Here's the drawing with two shaded views (mm, measured from the low corner). I have some questions. Coordinates: 2 decimals unless noted, no trailing zeros. Loops run counter-clockwise (first coordinate to the right, second up) from the corner with the lowest first, then second, coordinate; pieces in that order, holes last.
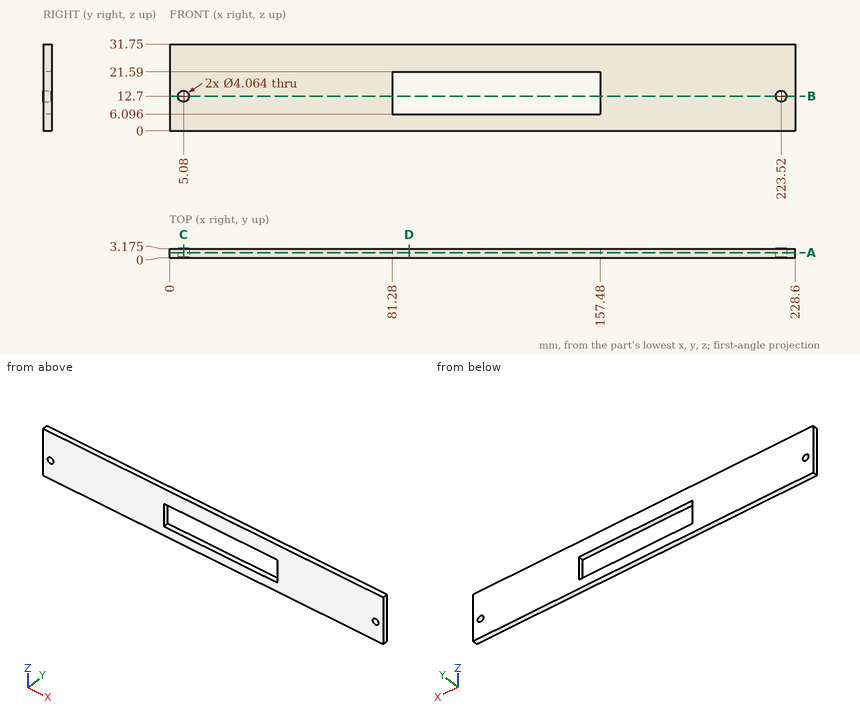
(1) I want a section at C-C on x = 5.08. Write out the boundary of the cut face in (y, z) (3 decimals).
Check values:
outline: (0, 0) - (3.175, 0) - (3.175, 10.668) - (0, 10.668) - close; (0, 14.732) - (3.175, 14.732) - (3.175, 31.75) - (0, 31.75) - close
(2) If I drill on probe 1 along X at (y, z) = (1.8, 12.7); probe 2 along Z at (x, y) = (223.52, 1.5); probe 3 along X at (y, z) = (2.6, 12.5), over which ranges is the centre line in solid material (lowest first)?
Check values:
probe 1: x = 0 to 3.05, 7.11 to 81.28, 157.48 to 221.49, 225.55 to 228.6
probe 2: z = 0 to 10.67, 14.73 to 31.75
probe 3: x = 0 to 3.06, 7.1 to 81.28, 157.48 to 221.5, 225.54 to 228.6
(3) I want a section at D-D on x = 87.5. Write out the boundary of the cut face in (y, z) (3 decimals), then the cut area to 3 significant figures.
Check values:
outline: (0, 0) - (3.175, 0) - (3.175, 6.096) - (0, 6.096) - close; (0, 21.59) - (3.175, 21.59) - (3.175, 31.75) - (0, 31.75) - close
area: 51.6 mm2
(4) I want a section at B-B on z = 12.7. Write out the boundary of the cut face in (x, y) (3 decimals).
Check values:
outline: (0, 0) - (3.048, 0) - (3.048, 3.175) - (0, 3.175) - close; (7.112, 0) - (81.28, 0) - (81.28, 3.175) - (7.112, 3.175) - close; (157.48, 0) - (221.488, 0) - (221.488, 3.175) - (157.48, 3.175) - close; (225.552, 0) - (228.6, 0) - (228.6, 3.175) - (225.552, 3.175) - close
(5) I want a section at A-A on y = 1.75. Write out the boundary of the cut face in (x, z).
Check values:
outline: (0, 0) - (228.6, 0) - (228.6, 31.75) - (0, 31.75) - close; hole circle Ø4.06 at (5.08, 12.7); hole (81.28, 6.1) - (157.48, 6.1) - (157.48, 21.59) - (81.28, 21.59) - close; hole circle Ø4.06 at (223.52, 12.7)
